```python
from build123d import *

# Parameters (mm, degrees)
SKETCH_W        = 76.2
SKETCH_H        = 76.2
PAD_DEPTH       = 4.5
SKETCH003_R     = 25.4
POCKET_DEPTH    = 4.501
SKETCH001_R     = 2.2
POCKET001_DEPTH = 4.501
SKETCH004_R     = 30.1625
POCKET002_DEPTH = 1.4


with BuildPart() as part:
    # Sketch → Pad (new body)
    with BuildSketch(Plane.XY):
        with Locations((38.1, 38.1)):
            Rectangle(SKETCH_W, SKETCH_H)
    extrude(amount=PAD_DEPTH)

    # Sketch003 (on Face6 of Pad) → Pocket (cut, through all)
    with BuildSketch(Plane.XY.offset(4.5)):
        with Locations((38.1, 38.1)):
            Circle(SKETCH003_R)
    extrude(amount=-POCKET_DEPTH, mode=Mode.SUBTRACT)

    # Sketch001 (on Face6 of Pad) → Pocket001 (cut, through all)
    with BuildSketch(Plane.XY.offset(4.5)):
        with Locations((8, 8)):
            Circle(SKETCH001_R)
        with Locations((68.2, 8)):
            Circle(SKETCH001_R)
        with Locations((68.2, 68.2)):
            Circle(SKETCH001_R)
        with Locations((8, 68.2)):
            Circle(SKETCH001_R)
    extrude(amount=-POCKET001_DEPTH, mode=Mode.SUBTRACT)

    # Sketch004 (on Face4 of Pocket001) → Pocket002 (cut)
    with BuildSketch(Plane(origin=(0, 0, 0), x_dir=(1, 0, 0), z_dir=(0, 0, -1))):
        with Locations((38.1, -38.1)):
            Circle(SKETCH004_R)
    extrude(amount=-POCKET002_DEPTH, mode=Mode.SUBTRACT)


solid = part.part
```
Model file for the job. Use its own axes, mm. A direction names the side the tool comes from. Give positions to 0.01 mm unless a question says otherwise; leave off trailing zeros. Loops run counter-clockwise (first coordinate to the right, second up) from the corner with the lowest first, then second, coordinate; pieces in that order, holes last. Notation, with made-up numbers: (32, -9) - (57, -9) arc R34 ccw to (57, 23) - close; hole circle Ø1 at (89.25, 21.5). An arc over 180 degrees is marked (long way). One line per item, written item: value. Start each with the question number.
1. Slice it at A-A (z = 3.5). List the corners of the cut face in (x, y).
2. Pull direction X, two halves, no side cores. Call faces 3 (the flat face through (12, 56, 0)), 4 (the flat face through (22, 58, 1.4)), 5 (the flat face through (76.2, 38, 2)): pulls with the +X half, pulls with the -X half, needs draft (parallel to the pull), parting line crosses it, or undercut.
3. Which spindle directions (+Z, -Z, +X, -X, +Y, -Y) get a long thin tool onto all of the face, cutting with end or side? Do faces 1 (the cylindrical face through (65.962, 49.652, 0.69)), 2 (the flat face through (12, 39, 4.5)). Say none if no direction does.
4. Slice it at D-D (y = 11.5). List the corners of the cut face in (x, z), plus the area to 3 significant figures.
5. Probe L1, parallel to Y at x = 68.2, z = 3.1; L2, parallel to X at y = 38.1, z = 1.1. List the from-to ranges inside material, lowest first. Write a range as from..to.
6. Slice it at B-B (x = 38.1). List the corners of the cut face in (y, z).
Solution:
1. outline: (0, 0) - (76.2, 0) - (76.2, 76.2) - (0, 76.2) - close; hole circle Ø4.4 at (8, 8); hole circle Ø4.4 at (8, 68.2); hole circle Ø50.8 at (38.1, 38.1); hole circle Ø4.4 at (68.2, 8); hole circle Ø4.4 at (68.2, 68.2)
2. face 3: needs draft
2. face 4: undercut
2. face 5: pulls with the +X half
3. face 1: -Z
3. face 2: +Z, +X, -X, +Y, -Y
4. outline: (0, 0) - (23.88, 0) - (23.88, 1.4) - (52.32, 1.4) - (52.32, 0) - (76.2, 0) - (76.2, 4.5) - (0, 4.5) - close
4. area: 303 mm^2
5. L1: y = 0..5.8, 10.2..66, 70.4..76.2
5. L2: x = 0..7.94, 68.26..76.2
6. outline: (0, 0) - (7.94, 0) - (7.94, 1.4) - (12.7, 1.4) - (12.7, 4.5) - (0, 4.5) - close; (63.5, 1.4) - (68.26, 1.4) - (68.26, 0) - (76.2, 0) - (76.2, 4.5) - (63.5, 4.5) - close
